Input: part model. Units: mm. Frame: model coordinates. Face numbers are marked on the shaded views. A direction names the side the tool comes from. Coordinates: 2 decimals unless noted, no trailing zeros. Loops run counter-clockwise (first coordinate to the right, second up) from the corner with the lowest first, then second, coordinate; pieces in that order, holes last. Notation, with made-up numbers: M 1.5,80.25 L 49.5,80.25 A22 cw 49.5,104.25 Z; hole C 48,30.25 d3. An arc over 180 degrees is marked long. Use a Markdown table: item, result. Add a question column.
1. Set-up query: the marked faces 1 and 2. Return all of +Z, -Z, +X, -X, +Y, -Y with unobstructed straight access to the full face (end or side cutting, diameter ignored); none if empty.
2. Section B-B on z = 0. Output: boundary loops of the cut face in (x, y).
3. Draft query along X for the marked faces 3, 4, 5 and 6. Return one class per face: +X half, -X half, draft (parallel to the pull), parting line (faces both ways), or undercut.
4. Pin query (flat end, axial travel): pin 1 (1.5 mm diameter, centred on x = -6, y = 1, fed in from +Z); pin 2 (4 mm diameter, centred on x = 23, z = -7.5, fed in from -Y); pin 3 (3 mm diameter, centred on y = 2, z = 18.5, fed in from -X). Return the tip coordinate at first contact, or that it passes through.
5. Line query: L1, parallel to X at y = 5, z = -18; L2, parallel to X at y = 13.5, z = 21; L3, parallel to Z at x = -19.5, y = 13.25. Output: solid intervals per line, ascending. Write a range as [from, to].
6. Section D-D on x = 21. Output: boundary loops of the cut face in (y, z), then the cut area to 3 significant figures.
7. Section A-A on x = 0. Output: boundary loops of the cut face in (y, z).
```python
from build123d import *

# Parameters (mm, degrees)
F0_R     = 19.05
F0_R_2   = 14.2875
F1_DEPTH = 7.9375
F2_R     = 30.1625
F3_DEPTH = 15.24
F4_R     = 6.35
F5_DEPTH = 23.1785
F6_R     = 32.385
F6_R_2   = 26.2509
F7_DEPTH = 12.7
F8_R     = 22.86
F9_DEPTH = 12.7


with BuildPart() as f1:
    # F0 (on Front) → F1 (new body)
    with BuildSketch(Plane.XZ):
        Circle(F0_R)
        Circle(F0_R_2, mode=Mode.SUBTRACT)
    extrude(amount=F1_DEPTH)

    # F2 (on face) → F3 (join)
    with BuildSketch(Plane(origin=(0, 0, 0), x_dir=(-1, 0, 0), z_dir=(0, 1, 0))):
        Circle(F2_R)
    extrude(amount=F3_DEPTH)

    # F4 (on face) → F5 (cut, through all)
    with BuildSketch(Plane(origin=(0, 15.24, 0), x_dir=(-1, 0, 0), z_dir=(0, 1, 0))):
        Circle(F4_R)
    extrude(amount=-F5_DEPTH, mode=Mode.SUBTRACT)

    # F6 (on face) → F7 (cut)
    with BuildSketch(Plane(origin=(0, 15.24, 0), x_dir=(-1, 0, 0), z_dir=(0, 1, 0))):
        Circle(F6_R)
        Circle(F6_R_2, mode=Mode.SUBTRACT)
    extrude(amount=-F7_DEPTH, mode=Mode.SUBTRACT)

    # F8 (on face) → F9 (cut)
    with BuildSketch(Plane(origin=(0, 15.24, 0), x_dir=(-1, 0, 0), z_dir=(0, 1, 0))):
        Circle(F8_R)
    extrude(amount=-F9_DEPTH, mode=Mode.SUBTRACT)


solid = f1.part
```
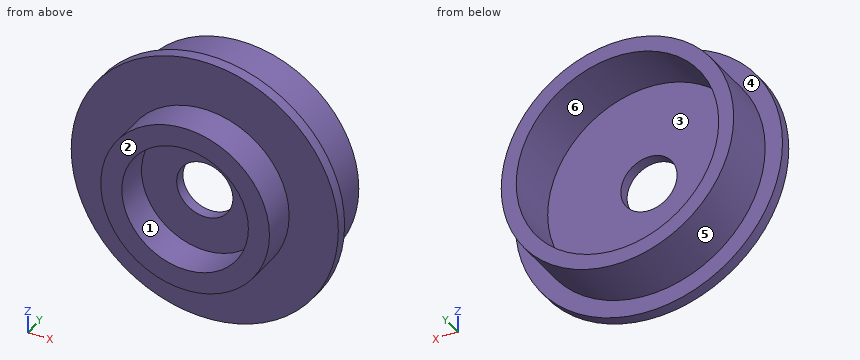
Answers below:
| question | item | result |
|---|---|---|
| 1 | face 1 | -Y |
| 1 | face 2 | +Z, -Z, +X, -X, -Y |
| 2 | outline | M -30.16,0 L -19.05,0 L -19.05,-7.94 L -14.29,-7.94 L -14.29,0 L -6.35,0 L -6.35,2.54 L -22.86,2.54 L -22.86,15.24 L -26.25,15.24 L -26.25,2.54 L -30.16,2.54 Z; M 6.35,0 L 14.29,0 L 14.29,-7.94 L 19.05,-7.94 L 19.05,0 L 30.16,0 L 30.16,2.54 L 26.25,2.54 L 26.25,15.24 L 22.86,15.24 L 22.86,2.54 L 6.35,2.54 Z |
| 3 | face 3 | undercut |
| 3 | face 4 | draft |
| 3 | face 5 | parting line |
| 3 | face 6 | undercut |
| 4 | pin 1 | stops at z = 29.7 |
| 4 | pin 2 | stops at y = 0 |
| 4 | pin 3 | stops at x = -24.92 |
| 5 | L1 | x = [-19.11, -14.09], [14.09, 19.11] |
| 5 | L2 | x = [-15.75, -9.03], [9.03, 15.75] |
| 5 | L3 | z = [-17.57, -11.93], [11.93, 17.57] |
| 6 | outline | M 0,-21.65 L 2.54,-21.65 L 2.54,-15.75 L 15.24,-15.75 L 15.24,-9.03 L 2.54,-9.03 L 2.54,9.03 L 15.24,9.03 L 15.24,15.75 L 2.54,15.75 L 2.54,21.65 L 0,21.65 Z |
| 6 | area | 281 mm² |
| 7 | outline | M -7.94,-19.05 L 0,-19.05 L 0,-30.16 L 2.54,-30.16 L 2.54,-26.25 L 15.24,-26.25 L 15.24,-22.86 L 2.54,-22.86 L 2.54,-6.35 L 0,-6.35 L 0,-14.29 L -7.94,-14.29 Z; M -7.94,14.29 L 0,14.29 L 0,6.35 L 2.54,6.35 L 2.54,22.86 L 15.24,22.86 L 15.24,26.25 L 2.54,26.25 L 2.54,30.16 L 0,30.16 L 0,19.05 L -7.94,19.05 Z |
